Model file for the job. Use its own axes, mm. Face numbers are marked on the shaded views. A direction names the side the tool comes from. Coordinates: 2 decimals unless noted, no trailing zeros. Order: outer loops, then holes, each group sorted by start corner. A loop starts at its lowest first (then second) coordinate and runs counter-clockwise, first axis right, second up.
from build123d import *

# Parameters (mm, degrees)
F0_R     = 10.3354497049
F1_DEPTH = 10


with BuildPart() as f1:
    # F0 (on Top) → F1 (new body)
    with BuildSketch(Plane.XY):
        with BuildLine():
            ThreePointArc((26.0476715205, -9.5277688633), (20.5866821195, -7.4048691039), (16.5865343387, -3.1237563563))
            ThreePointArc((16.5865343387, -3.1237563563), (16.6143313263, 1.8736112558), (20.9546162977, 4.350783452))
            Line((20.9546162977, 4.350783452), (35.7516345046, 4.2815737703))
            ThreePointArc((35.7516345046, 4.2815737703), (38.1912718914, 3.6328944013), (40.0030732107, 1.875057241))
            ThreePointArc((40.0030732107, 1.875057241), (59.6888453726, 3.3154186125), (46.9838539695, 18.4212936265))
            ThreePointArc((46.9838539695, 18.4212936265), (43.7332768295, 18.7671729362), (41.391113059, 21.0475573584))
            ThreePointArc((41.391113059, 21.0475573584), (30.4913773374, 35.1718790284), (15.1030881654, 44.199683734))
            ThreePointArc((15.1030881654, 44.199683734), (13.3602329953, 45.2544090168), (12.1827503516, 46.9167941077))
            ThreePointArc((12.1827503516, 46.9167941077), (-8.7169198304, 51.6376390641), (-6.9602796681, 30.2835573428))
            ThreePointArc((-6.9602796681, 30.2835573428), (-5.9948536036, 29.5104843528), (-5.2487236207, 28.52408718))
            Line((-5.2487236207, 28.52408718), (-4.5951623795, 27.3920859044))
            ThreePointArc((-4.5951623795, 27.3920859044), (-3.9403401472, 25.2797467908), (-4.2607272631, 23.0915692881))
            Line((-4.2607272631, 23.0915692881), (-6.3719962821, 17.6219471616))
            ThreePointArc((-6.3719962821, 17.6219471616), (-10.6605564778, 14.4366215681), (-15.3783311249, 16.9427440847))
            Line((-15.3783311249, 16.9427440847), (-21.8734443287, 28.3151202921))
            ThreePointArc((-21.8734443287, 28.3151202921), (-22.531440873, 30.8428756983), (-21.8249990194, 33.3575221452))
            ThreePointArc((-21.8249990194, 33.3575221452), (-32.3826009658, 50.070876996), (-39.625901643, 31.6770251828))
            ThreePointArc((-39.625901643, 31.6770251828), (-38.3773400055, 28.7239903076), (-39.1790717552, 25.619711432))
            ThreePointArc((-39.1790717552, 25.619711432), (-45.9266907543, 9.0613660016), (-45.9738489372, -8.8189847124))
            ThreePointArc((-45.9738489372, -8.8189847124), (-46.0225178396, -10.9283689132), (-46.9369511167, -12.8298636279))
            ThreePointArc((-46.9369511167, -12.8298636279), (-40.8714994553, -33.5184892265), (-23.1566713845, -21.2305357989))
            ThreePointArc((-23.1566713845, -21.2305357989), (-23.0733624914, -20.408634033), (-22.8558581112, -19.6116680808))
            ThreePointArc((-22.8558581112, -19.6116680808), (-20.2416339534, -17.248733359), (-16.9474626281, -15.9973086803))
            Line((-16.9474626281, -15.9973086803), (-12.5698108847, -15.2138142303))
            ThreePointArc((-12.5698108847, -15.2138142303), (-7.5901456855, -17.2720461747), (-7.3705416357, -22.6558327877))
            Line((-7.3705416357, -22.6558327877), (-13.4673451749, -33.1026572937))
            ThreePointArc((-13.4673451749, -33.1026572937), (-15.3433779099, -34.9453329591), (-17.8949610773, -35.5812384318))
            ThreePointArc((-17.8949610773, -35.5812384318), (-27.1947516812, -53.0465292991), (-7.6201577031, -50.1555500621))
            ThreePointArc((-7.6201577031, -50.1555500621), (-5.6870353017, -47.5977465283), (-2.5977850601, -46.7399271527))
            ThreePointArc((-2.5977850601, -46.7399271527), (14.979861549, -44.3505696179), (30.4063859475, -35.5924285638))
            ThreePointArc((30.4063859475, -35.5924285638), (32.226193311, -34.6022844585), (34.2911475267, -34.4348082622))
            ThreePointArc((34.2911475267, -34.4348082622), (49.1043559344, -19.1319266108), (30.223953434, -9.2759775653))
            ThreePointArc((30.223953434, -9.2759775653), (28.8084467622, -9.7132375899), (27.326945928, -9.7165155971))
            Line((27.326945928, -9.7165155971), (26.0476715205, -9.5277688633))
        make_face()
        Polygon((-25.6983195519, -48.8112031808), (-23.1400125477, -41.0882104714), (-15.1725511659, -39.442272973), (-9.7633967884, -45.5193281841), (-12.3217037926, -53.2423208936), (-20.2891651744, -54.888258392), align=None, mode=Mode.SUBTRACT)
        Polygon((-25.6526473767, -17.6703529021), (-28.1761860468, -28.6749401878), (-38.9682075294, -31.991785235), (-47.2366903419, -24.3040429964), (-44.7131516719, -13.2994557107), (-33.9211301893, -9.9826106636), align=None, mode=Mode.SUBTRACT)
        with BuildLine():
            ThreePointArc((17.1464472205, -14.3181778051), (19.6097516752, -15.0995212956), (21.4092604692, -16.9542812764))
            Line((21.4092604692, -16.9542812764), (22.0381273172, -18.0435106083))
            ThreePointArc((22.0381273172, -18.0435106083), (22.5618213465, -19.3433351078), (22.7042381867, -20.7374357532))
            ThreePointArc((22.7042381867, -20.7374357532), (23.1173853103, -24.5798156567), (24.6184803157, -28.1408952196))
            ThreePointArc((24.6184803157, -28.1408952196), (25.2428792275, -31.7249542816), (23.2729013133, -34.7834735932))
            ThreePointArc((23.2729013133, -34.7834735932), (9.419684867, -41.2411709688), (-5.8406517441, -42.0988351334))
            ThreePointArc((-5.8406517441, -42.0988351334), (-7.725446025, -41.4431302055), (-9.2036800008, -40.1025248397))
            ThreePointArc((-9.2036800008, -40.1025248397), (-9.295625501, -39.9790891343), (-9.3892764279, -39.8569422871))
            ThreePointArc((-9.3892764279, -39.8569422871), (-10.4294976001, -37.1481783868), (-9.7902204963, -34.3178450603))
            Line((-9.7902204963, -34.3178450603), (0.5477905756, -16.116209429))
            ThreePointArc((0.5477905756, -16.116209429), (2.5119825197, -14.1902261445), (5.1976512462, -13.5947052828))
            Line((5.1976512462, -13.5947052828), (17.1464472205, -14.3181778051))
        make_face(mode=Mode.SUBTRACT)
        with BuildLine():
            Line((16.6011031737, -3.1491618567), (16.5626926236, -3.0826328324))
            ThreePointArc((16.5626926236, -3.0826328324), (16.574594931, -3.103205349), (16.5865343387, -3.1237563563))
            ThreePointArc((16.5865343387, -3.1237563563), (16.5938001553, -3.1364697732), (16.6011031737, -3.1491618567))
        make_face(mode=Mode.SUBTRACT)
        Polygon((44.4996077616, -28.8073727903), (33.6737244283, -32.1346250176), (25.3656168325, -23.8068915105), (27.8220380789, -13.0949882861), (38.8145774711, -9.7165155971), (47.2366903419, -17.5470976183), (44.7015978404, -28.6020685768), (44.6662638205, -28.7561523286), align=None, mode=Mode.SUBTRACT)
        with BuildLine():
            ThreePointArc((-17.8096832999, -5.2424840404), (-21.2796968224, -8.7124975629), (-26.0198234456, -9.9826106636))
            Line((-26.0198234456, -9.9826106636), (-27.5911085786, -9.9826106636))
            ThreePointArc((-27.5911085786, -9.9826106636), (-28.8409335841, -9.8238850264), (-30.0114068814, -9.3577856459))
            ThreePointArc((-30.0114068814, -9.3577856459), (-33.2357643816, -8.090181928), (-36.6781903014, -7.6990243375))
            ThreePointArc((-36.6781903014, -7.6990243375), (-40.152524922, -6.3783493463), (-41.7554658188, -3.0248789097))
            ThreePointArc((-41.7554658188, -3.0248789097), (-39.9512896461, 12.2753331327), (-32.80623714, 25.9245003194))
            ThreePointArc((-32.80623714, 25.9245003194), (-28.5358777475, 27.8291904256), (-24.5583425883, 25.3709333601))
            Line((-24.5583425883, 25.3709333601), (-13.7204299658, 6.9015986867))
            ThreePointArc((-13.7204299658, 6.9015986867), (-13.0328237883, 4.3887357815), (-13.7026655941, 1.8710792937))
            Line((-13.7026655941, 1.8710792937), (-17.8096832999, -5.2424840404))
        make_face(mode=Mode.SUBTRACT)
        Circle(F0_R, mode=Mode.SUBTRACT)
        Polygon((-23.6072220849, 40.0795913092), (-26.1655290892, 32.3565985997), (-34.132990471, 30.7106611014), (-39.5421448485, 36.7877163125), (-36.9838378442, 44.510709022), (-29.0163764624, 46.1566465203), align=None, mode=Mode.SUBTRACT)
        Polygon((2.5704265214, 53.060195325), (10.9925393922, 45.2296133038), (8.4221128708, 34.0205585935), (-2.5704265214, 30.6420859044), (-10.9925393922, 38.4726679257), (-8.4221128708, 49.6817226359), align=None, mode=Mode.SUBTRACT)
        with BuildLine():
            ThreePointArc((4.3285128423, 20.4325643906), (3.6004962361, 23.9453268817), (4.5951623795, 27.3920859044))
            Line((4.5951623795, 27.3920859044), (5.2487236207, 28.52408718))
            ThreePointArc((5.2487236207, 28.52408718), (5.9948536036, 29.5104843528), (6.9602796681, 30.2835573428))
            ThreePointArc((6.9602796681, 30.2835573428), (9.71050055, 32.5314875149), (11.7670884139, 35.4275799367))
            ThreePointArc((11.7670884139, 35.4275799367), (14.6903203036, 37.8718936539), (18.4869211069, 37.5466605538))
            ThreePointArc((18.4869211069, 37.5466605538), (30.8412464649, 28.1036186684), (39.1761724906, 14.9761892458))
            ThreePointArc((39.1761724906, 14.9761892458), (38.7132835477, 10.307822352), (34.5859321139, 8.0778255422))
            Line((34.5859321139, 8.0778255422), (13.5057011722, 7.9289416207))
            ThreePointArc((13.5057011722, 7.9289416207), (10.8213953927, 8.6881995171), (8.9616649904, 10.7674717221))
            Line((8.9616649904, 10.7674717221), (4.3285128423, 20.4325643906))
        make_face(mode=Mode.SUBTRACT)
        with BuildLine():
            Line((54.8872223768, 1.5462432454), (46.919760995, -0.099694253))
            ThreePointArc((46.919760995, -0.099694253), (46.8658270284, -0.0816186896), (46.8120207581, -0.0631664804))
            ThreePointArc((46.8120207581, -0.0631664804), (46.8120586965, -0.020929805), (46.8120585264, 0.0213068875))
            Line((46.8120585264, 0.0213068875), (41.5106066175, 5.9773609582))
            Line((41.5106066175, 5.9773609582), (44.0689136218, 13.7003536676))
            Line((44.0689136218, 13.7003536676), (52.0363750036, 15.346291166))
            Line((52.0363750036, 15.346291166), (57.4455293811, 9.2692359549))
            Line((57.4455293811, 9.2692359549), (54.8872223768, 1.5462432454))
        make_face(mode=Mode.SUBTRACT)
        with BuildLine():
            ThreePointArc((16.5865343387, -3.1237563563), (16.574594931, -3.103205349), (16.5626926236, -3.0826328324))
            Line((16.5626926236, -3.0826328324), (16.6011031737, -3.1491618567))
            ThreePointArc((16.6011031737, -3.1491618567), (16.5938001553, -3.1364697732), (16.5865343387, -3.1237563563))
        make_face()
    extrude(amount=F1_DEPTH)


solid = f1.part
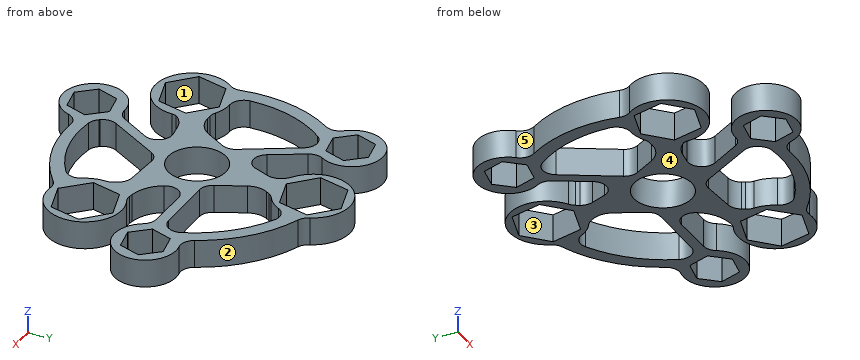
Q1. Mould opens along X. For the marked faces 3, 4 and 5 say: pulls with the +X half, pulls with the -X half, needs draft (parallel to the pull), parting line crosses it, or undercut.
Established:
face 3: undercut
face 4: needs draft
face 5: pulls with the -X half
Q2. Cut at A-A, the plane y = -37. List the corners of the cut face in (x, z), plus the area to 3 significant figures.
Established:
outline: (-23.57, 0) - (-10.44, 0) - (-10.44, 10) - (-23.57, 10) - close; (19.86, 0) - (28.68, 0) - (28.68, 10) - (19.86, 10) - close
area: 219 mm2
Q3. Cut at B-B, the plane z = 4.5. Count the separate pieces of the cut face and the enclosed holes in it, plus the area to 3 significant figures.
Established:
separate pieces: 1
enclosed holes: 10
area: 3,040 mm2
Q4. Which spindle directions (+Z, -Z, +X, -X, +Y, -Y) get a long thin tool onto all of the face, cutting with end or side? Do the marked faces 1 and 2. Say none if no direction does.
Established:
face 1: +Z, -Z
face 2: +Z, -Z, +X, +Y
Q5. Drop flat-ended pins along their axis: P1, Ø18.5, axis at x = 0, y = 0, coming from the +Z side; P2, Ø1.5, axis at y = -2.5, z = 3.5, coming from the -X side; P3, Ø1.5, axis at y = -46, z = 8.5, coming from the -X side; P4, Ø5, axis at y = 16, z = 2, coming from the +X side. Give the stop position or say it passes through.
Established:
P1: passes through
P2: stops at x = -46.78
P3: stops at x = -29.22
P4: stops at x = 58.87
Q6. Probe line 1 (Y direction, x = 0, z = 2.5); line 2 (X direction, y = -19, z = 5); line 3 (Y direction, x = 38, z = 1.25). List the from-to ranges inside material, lowest first.
Established:
line 1: y = -46.81 to -42.46, -17.08 to -10.34, 10.34 to 31.43, 52.27 to 54.9
line 2: x = -49.59 to -46.02, -25.96 to -22.35, -6.82 to -1.09, 22.46 to 26.47, 46.9 to 49.08
line 3: y = -34.39 to -30.8, -9.97 to -8.12, 3.74 to 9.46, 17.6 to 26.75
